from build123d import *

# Parameters (mm, degrees)
CROQUIS1_W                 = 60
CROQUIS1_H                 = 60
SALIENTE_EXTRUIR1_DEPTH    = 3
CROQUIS2_W                 = 40
CROQUIS2_H                 = 40
CROQUIS2_W_2               = 30
CROQUIS2_H_2               = 30
SALIENTE_EXTRUIR2_DEPTH    = 30
CHAFL_N1_SIZE              = 3
REDONDEO1_R                = 3
CROQUIS3_R                 = 1.5
CORTAR_EXTRUIR1_DEPTH      = 30
CORTAR_EXTRUIR2_DEPTH      = 54.749418602
CORTAR_EXTRUIR2_DEPTH_BACK = 54.749418602
CROQUIS4_R                 = 3


with BuildPart() as part:
    # Croquis1 → Saliente-Extruir1 (new body)
    with BuildSketch(Plane(origin=(0, 0, 0), x_dir=(1, 0, 0), z_dir=(0, 1, 0))):
        Rectangle(CROQUIS1_W, CROQUIS1_H)
    extrude(amount=SALIENTE_EXTRUIR1_DEPTH)

    # Croquis2 → Saliente-Extruir2 (add)
    with BuildSketch(Plane(origin=(0, 3, 0), x_dir=(1, 0, 0), z_dir=(0, 1, 0))):
        Rectangle(CROQUIS2_W, CROQUIS2_H)
        Rectangle(CROQUIS2_W_2, CROQUIS2_H_2, mode=Mode.SUBTRACT)
    extrude(amount=SALIENTE_EXTRUIR2_DEPTH)

    # Chaflán1
    chafl_n1_edges = [part.edges().sort_by_distance(p)[0] for p in [
        (0, 33, 20),
        (20, 33, 0),
        (0, 33, -20),
        (-20, 33, 0),
    ]]
    chamfer(chafl_n1_edges, length=CHAFL_N1_SIZE)

    # Redondeo1
    redondeo1_edges = [part.edges().sort_by_distance(p)[0] for p in [
        (0, 3, 20),
        (20, 3, 0),
        (0, 3, -20),
        (-20, 3, 0),
    ]]
    fillet(redondeo1_edges, radius=REDONDEO1_R)

    # Croquis3 → Cortar-Extruir1 (cut)
    with BuildSketch(Plane(origin=(0, 3, 0), x_dir=(1, 0, 0), z_dir=(0, 1, 0))):
        with Locations(Location((0, 26.5, 0), (0, 0, 270))):
            Circle(CROQUIS3_R)
        with Locations(Location((15, 26.5, 0), (0, 0, 270))):
            Circle(CROQUIS3_R)
        with Locations(Location((-15, 26.5, 0), (0, 0, 90))):
            Circle(CROQUIS3_R)
        with Locations(Location((26.5, 15, 0), (0, 0, 90))):
            Circle(CROQUIS3_R)
        with Locations(Location((26.5, 0, 0), (0, 0, 270))):
            Circle(CROQUIS3_R)
        with Locations(Location((26.5, -15, 0), (0, 0, 270))):
            Circle(CROQUIS3_R)
        with Locations(Location((15, -26.5, 0), (0, 0, 90))):
            Circle(CROQUIS3_R)
        with Locations(Location((0, -26.5, 0), (0, 0, 270))):
            Circle(CROQUIS3_R)
        with Locations(Location((-15, -26.5, 0), (0, 0, 270))):
            Circle(CROQUIS3_R)
        with Locations(Location((-26.5, -15, 0), (0, 0, 90))):
            Circle(CROQUIS3_R)
        with Locations(Location((-26.5, 0, 0), (0, 0, 270))):
            Circle(CROQUIS3_R)
        with Locations(Location((-26.5, 15, 0), (0, 0, 270))):
            Circle(CROQUIS3_R)
    extrude(amount=-CORTAR_EXTRUIR1_DEPTH, mode=Mode.SUBTRACT)

    # Croquis4 → Cortar-Extruir2 (cut, two sides: drawn at the far end of the back side and taken through both)
    with BuildSketch(Plane(origin=(0, 0, 0), x_dir=(0, 0, -1), z_dir=(1, 0, 0)).offset(-CORTAR_EXTRUIR2_DEPTH_BACK)):
        with Locations((0, 20)):
            Circle(CROQUIS4_R)
    extrude(amount=CORTAR_EXTRUIR2_DEPTH + CORTAR_EXTRUIR2_DEPTH_BACK, mode=Mode.SUBTRACT)


solid = part.part
Geometry: final body of the model. Coordinates: model frame, mm. A direction names the side the tool comes from. Give positions to 0.01 mm unless a question says otherwise; leave off trailing zeros. Write each loop counter-clockwise with the first axis right and the second up, starting at its lowest first coordinate (ties: lowest second). Pieces come first, ordered by that corner, then holes. Notation, with made-up numbers: (29.5, 64.5) - (35.5, 64.5) arc R17 cw to (35.5, 74.5) - close; hole circle Ø3 at (-1.5, -25.75). An arc over 180 degrees is marked (long way). Return JSON: item names as keys, results as strings. Group by question number.
1) Mould query, pull axis Z, two halves, no side actions, for faces 1 (the flat face through (0, 32, 18)), 2 (the cylindrical face through (0, 2, 25)), 3 (the flat face through (-18, 32, 0)). Classes: released by +Z, released by -Z, zero draft, split by the parting line, or undercut.
2) Section A-A on y = 2. State how many separate pieces and enclosed holes the cut face has, plus the area to 3 significant figures.
3) Section D-D on y = 20. Return the cut outline in (x, z).
4) First-contact query: P1, Ø6, axis at x = -9, z = 7.5, coming from the +Y side; P2, Ø19, axis at y = 17.5, z = 7, coming from the +X side; P3, Ø10, axis at x = 12, y = 25.5, coming from the -Z side. Flat tips, straight axial feed; report the tip coordinate or a pass-through.
5) Set-up query: faces 4 (the cylindrical face through (0.32, 3.9, 20.86)), 5 (the flat face through (15, 14, 0)), 6 (the flat face through (-20, 15, 0)). Return all of +Z, -Z, +X, -X, +Y, -Y with unobstructed straight access to the full face (end or side cutting, diameter ignored); none if empty.
6) Line query: line 1 (X direction, y = 1.4, z = 0); line 2 (X direction, y = 0.8, z = -26.5); line 3 (Z direction, x = 12, y = 27). Output: solid intervals per line, ascending.
7) Section B-B on z = -26.5. Return the cut outline in (x, y).
Filled in:
{
 "1": {"face 1": "released by +Z", "face 2": "undercut", "face 3": "zero draft"},
 "2": {"separate pieces": "1", "enclosed holes": "12", "area": "3,520 mm^2"},
 "3": {"outline": "(-20, -20) - (20, -20) - (20, -3) - (15, -3) - (15, -15) - (-15, -15) - (-15, -3) - (-20, -3) - close; (-20, 3) - (-15, 3) - (-15, 15) - (15, 15) - (15, 3) - (20, 3) - (20, 20) - (-20, 20) - close"},
 "4": {"P1": "stops at y = 3", "P2": "stops at x = 20", "P3": "stops at z = -20"},
 "5": {"face 4": "+Z, +X, -X, +Y", "face 5": "+Y", "face 6": "+Z, -Z, -X, +Y"},
 "6": {"line 1": "x = -30 to -28, -25 to 25, 28 to 30", "line 2": "x = -30 to -16.5, -13.5 to -1.5, 1.5 to 13.5, 16.5 to 30", "line 3": "z = -20 to -15, 15 to 20"},
 "7": {"outline": "(-30, 0) - (-16.5, 0) - (-16.5, 3) - (-30, 3) - close; (-13.5, 0) - (-1.5, 0) - (-1.5, 3) - (-13.5, 3) - close; (1.5, 0) - (13.5, 0) - (13.5, 3) - (1.5, 3) - close; (16.5, 0) - (30, 0) - (30, 3) - (16.5, 3) - close"}
}
